Source: CAD feature listing. Evaluate the final solid. Frame: model axes, mm. A direction names the side the tool comes from. Give positions to 0.01 mm unless a question says otherwise; leave off trailing zeros. Order: outer loops, then holes, each group sorted by start corner. A loop starts at its lowest first (then second) coordinate and runs counter-clockwise, first axis right, second up. Notation, with made-up numbers: (7.25, 45.25) -> (38.25, 45.25) arc R5 cw to (38.25, 49.25) -> close; hole circle Ø4 at (1, 18). An arc over 180 degrees is marked (long way). Answer in a Markdown table with one row per item.
```python
from build123d import *

# Parameters (mm, degrees)
EXTRUDE1_DEPTH         = 127
SKETCH2_R              = 6.731
CUT_CHAMFER_DEPTH      = 508
CUT_CHAMFER_DEPTH_BACK = 58.15
SKETCH3_R              = 6.731
CUT_HOLES_DEPTH        = 229.6


with BuildPart() as part:
    # Sketch1 → Extrude1 (new body, symmetric)
    with BuildSketch(Plane.XY):
        with BuildLine():
            Line((228.6, 0), (15.875, 0))
            ThreePointArc((15.875, 0), (4.649679849, -4.649679849), (0, -15.875))
            Line((0, -15.875), (0, -57.15))
            Line((0, -57.15), (6.35, -57.15))
            Line((6.35, -57.15), (6.35, -15.875))
            ThreePointArc((6.35, -15.875), (9.139807909, -9.139807909), (15.875, -6.35))
            Line((15.875, -6.35), (228.6, -6.35))
            Line((228.6, -6.35), (228.6, 0))
        make_face()
    extrude(amount=EXTRUDE1_DEPTH, both=True)

    # Sketch2 → Cut-Chamfer (cut, two sides)
    with BuildSketch(Plane(origin=(0, 0, 0), x_dir=(1, 0, 0), z_dir=(0, 1, 0))) as cut_chamfer_sk:
        with Locations((209.55, 38.1)):
            Circle(SKETCH2_R)
        with Locations((139.7, 38.1)):
            Circle(SKETCH2_R)
        with Locations((209.55, 0)):
            Circle(SKETCH2_R)
        with Locations((139.7, 0)):
            Circle(SKETCH2_R)
        with Locations((139.7, -38.1)):
            Circle(SKETCH2_R)
        with Locations((209.55, -38.1)):
            Circle(SKETCH2_R)
        Polygon((25.4, 127), (228.6, 53.975), (228.6, 127), align=None)
        Polygon((228.6, -53.975), (228.6, -127), (25.4, -127), align=None)
    extrude(amount=CUT_CHAMFER_DEPTH, mode=Mode.SUBTRACT)
    extrude(cut_chamfer_sk.sketch, amount=-CUT_CHAMFER_DEPTH_BACK, mode=Mode.SUBTRACT)

    # Sketch3 → Cut-Holes (cut, through all)
    with BuildSketch(Plane(origin=(0, 0, 0), x_dir=(0, 0, -1), z_dir=(1, 0, 0))):
        with Locations((0, -36.5125)):
            Circle(SKETCH3_R)
        with Locations((101.6, -36.5125)):
            Circle(SKETCH3_R)
        with Locations((0, -150.8125)):
            Circle(SKETCH3_R)
        with Locations((101.6, -150.8125)):
            Circle(SKETCH3_R)
        with Locations((-101.6, -36.5125)):
            Circle(SKETCH3_R)
        with Locations((-101.6, -150.8125)):
            Circle(SKETCH3_R)
        with Locations((-50.8, -36.5125)):
            Circle(SKETCH3_R)
        with Locations((50.8, -36.5125)):
            Circle(SKETCH3_R)
        with Locations((50.8, -150.8125)):
            Circle(SKETCH3_R)
        with Locations((-50.8, -150.8125)):
            Circle(SKETCH3_R)
    extrude(amount=CUT_HOLES_DEPTH, mode=Mode.SUBTRACT)


solid = part.part
```
(1) Pull-direction query (X, two-part tool) for faces 1 (the flat face through (228.6, -3, 1)), 2 (the cylindrical face through (215.97, -3.13, -2.02)), 3 (the flat face through (6, -24, 127)); classes: +X half, -X half, draft (parallel to the pull), parting line (faces both ways), or undercut.
A:
| item | result |
|---|---|
| face 1 | +X half |
| face 2 | undercut |
| face 3 | draft |
(2) Section query B-B (x = 139.7). Return the cut outline in (y, z), plus the area to 3 significant figures.
A:
| item | result |
|---|---|
| outline | (-6.35, -85.92) -> (0, -85.92) -> (0, -44.83) -> (-6.35, -44.83) -> close; (-6.35, -31.37) -> (0, -31.37) -> (0, -6.73) -> (-6.35, -6.73) -> close; (-6.35, 6.73) -> (0, 6.73) -> (0, 31.37) -> (-6.35, 31.37) -> close; (-6.35, 44.83) -> (0, 44.83) -> (0, 85.92) -> (-6.35, 85.92) -> close |
| area | 835 mm^2 |
(3) Section query C-C (z = 20.5). Return the cut outline in (x, y) (3 decimals), plus the area to 3 significant figures.
A:
| item | result |
|---|---|
| outline | (0, -57.15) -> (6.35, -57.15) -> (6.35, -15.875) arc R9.525 cw to (15.875, -6.35) -> (228.6, -6.35) -> (228.6, 0) -> (15.875, 0) arc R15.875 ccw to (0, -15.875) -> close |
| area | 1,740 mm^2 |
(4) Ray query, probe 1 along Z at (x, y) = (139, -4) (1 decimal); probe 2 along Z at (x, y) = (209, -1); probe 3 along X at (y, z) = (-24.5, -93.5). Return the intervals inside material, ascending.
A:
| item | result |
|---|---|
| probe 1 | z = -86.2 to -44.8, -31.4 to -6.7, 6.7 to 31.4, 44.8 to 86.2 |
| probe 2 | z = -61.02 to -44.81, -31.39 to -6.71, 6.71 to 31.39, 44.81 to 61.02 |
| probe 3 | x = 0 to 6.35 |
(5) First-contact query: pin 1 Ø10 at (y, z) = (-38.5, 36.5) entering from +X; pin 2 Ø15.5 at (x, z) = (139.7, 38.1) entering from -Y. Flat tips, straight axial feed; report the tip coordinate or a pass-through.
A:
| item | result |
|---|---|
| pin 1 | stops at x = 6.35 |
| pin 2 | stops at y = -6.35 |
(6) Section query D-D (y = -22). Return the cut outline in (x, z), plus the area to 3 significant figures.
A:
| item | result |
|---|---|
| outline | (0, -127) -> (6.35, -127) -> (6.35, 127) -> (0, 127) -> close |
| area | 1,610 mm^2 |
(7) Access query for faces 4 (the flat face through (97, -6.35, 2)), 5 (the cylindrical face through (134.36, -3.13, 42.2)). Directions: +Z, -Z, +X, -X, +Y, -Y. A direction counts if a zero-diameter tool reaches every point of the face in a straight line with its end or side. Return the directions, or none.
A:
| item | result |
|---|---|
| face 4 | +Z, -Z, +X, -Y |
| face 5 | +Y, -Y |
